from build123d import *

# Parameters (mm, degrees)
SKETCH1_R           = 0.4445
BOSS_EXTRUDE1_DEPTH = 1
SKETCH2_R           = 0.127
BOSS_EXTRUDE2_DEPTH = 12.7
SKETCH3_R           = 0.127
CIRPATTERN1_COUNT   = 6


with BuildPart() as part:
    # Sketch1 → Boss-Extrude1 (new body)
    with BuildSketch(Plane(origin=(0, 0, 0), x_dir=(1, 0, 0), z_dir=(0, 1, 0))):
        with Locations(Location((0, 0, 0), (0, 0, 270))):
            Circle(SKETCH1_R)
    extrude(amount=BOSS_EXTRUDE1_DEPTH)

    # Sketch2 → Boss-Extrude2 (add)
    with BuildSketch(Plane(origin=(0, 1, 0), x_dir=(1, 0, 0), z_dir=(0, 1, 0))):
        with Locations(Location((0, 0, 0), (0, 0, 270))):
            Circle(SKETCH2_R)
    extrude(amount=BOSS_EXTRUDE2_DEPTH)

    # Sweep2: sweep along a curve in space
    with BuildLine() as sweep2_path:
        Line((0, 1, -0.3048), (0, 2.789892119, -1.512097479))
    # Sketch3 → Sweep2 (sweep)
    with BuildSketch(Plane(origin=(0, 1, 0), x_dir=(1, 0, 0), z_dir=(0, 1, 0))):
        with Locations((0, 0.3048)):
            Circle(SKETCH3_R)
    sweep2 = sweep(path=sweep2_path.line)

    # CirPattern1: Sweep2 ×6 about axis
    cirpattern1_axis = Axis((0, 1, 0), (0, 1, 0))
    for i in range(1, CIRPATTERN1_COUNT):
        add(sweep2.rotate(cirpattern1_axis, i * 360 / CIRPATTERN1_COUNT))


solid = part.part
Input: part model. Units: mm. Frame: model coordinates. A direction names the side the tool comes from. Give positions to 0.01 mm unless a question says otherwise; leave off trailing zeros. Order: outer loops, then holes, each group sorted by start corner. A loop starts at its lowest first (then second) coordinate and runs counter-clockwise, first axis right, second up. Notation, with made-up numbers: (12, -27) - (29, -27) arc R12 cw to (29, -17) - close; hole circle Ø7 at (80.5, 17). An arc over 180 degrees is marked (long way). Answer as a JSON object with one key per item and string values. Group by question number.
Q1. Set-up query: faces 1 (the face through (0, 0, 0)), 2 (the face through (-0.434, 0.493, -0.096)). Return all of +Z, -Z, +X, -X, +Y, -Y with unobstructed straight access to the full face (end or side cutting, diameter ignored); none if empty.
Q2. First-contact query: pin 1 Ø1 at (y, z) = (4, 1) entering from -X; pin 2 Ø1.5 at (x, z) = (-0.5, -1) entering from +Y. Flat tips, straight axial feed; report the tip coordinate or a pass-through.
Q3. Cut plane A-A, the plane y = 10. Output: boundary loops of the cut face in (x, z).
Q4. Cut plane B-B, the plane y = 1.25. Count the separate pieces of the cut face and the enclosed holes in it, then the cut area to 3 significant figures.
Q5. Line query: probe 1 along Z at (x, y) = (-0.05, 2.25); probe 2 along Y at (x, z) = (-0.05, -1.05); probe 3 along Z at (x, y) = (0.05, 10). Output: solid intervals per line, ascending.
Results:
{
 "1": {"face 1": "+Z, -Z, +X, -X, -Y", "face 2": "-Y"},
 "2": {"pin 1": "through", "pin 2": "y = 2.79"},
 "3": {"outline": "circle Ø0.25 at (0, 0)"},
 "4": {"separate pieces": "7", "enclosed holes": "0", "area": "0.355 mm^2"},
 "5": {"probe 1": "-1.26 to -1.03, -0.12 to 0.12, 1.03 to 1.26", "probe 2": "1.93 to 2.28", "probe 3": "-0.12 to 0.12"}
}
